```python
from build123d import *

# Parameters (mm, degrees)
SKETCH2_W           = 20
SKETCH2_H           = 10
BOSS_EXTRUDE1_DEPTH = 110
CUT_EXTRUDE1_DEPTH  = 10
SKETCH5_W           = 10
SKETCH5_H           = 60
CUT_EXTRUDE2_DEPTH  = 10
BOSS_EXTRUDE2_DEPTH = 10
FILLET1_R           = 1


with BuildPart() as part:
    # Sketch2 → Boss-Extrude1 (new body)
    with BuildSketch(Plane(origin=(0, 0, 0), x_dir=(1, 0, 0), z_dir=(0, 1, 0))):
        Rectangle(SKETCH2_W, SKETCH2_H)
    extrude(amount=BOSS_EXTRUDE1_DEPTH)

    # Sketch3 → Cut-Extrude1 (cut)
    with BuildSketch(Plane.XY.offset(5)):
        with BuildLine():
            Line((-4.9, 110), (-4.9, 95))
            ThreePointArc((-4.9, 95), (0, 90.1), (4.9, 95))
            Line((4.9, 95), (4.9, 110))
            Line((4.9, 110), (-4.9, 110))
        make_face()
    extrude(amount=-CUT_EXTRUDE1_DEPTH, mode=Mode.SUBTRACT)

    # Sketch5 → Cut-Extrude2 (cut)
    with BuildSketch(Plane.XY.offset(5)):
        with BuildLine():
            Line((-5, 15.05), (5, 15.05))
            ThreePointArc((5, 15.05), (0, 10.05), (-5, 15.05))
        make_face()
        with Locations((0, 45.05)):
            Rectangle(SKETCH5_W, SKETCH5_H)
        with BuildLine():
            ThreePointArc((-5, 75.05), (0, 80.05), (5, 75.05))
            Line((5, 75.05), (-5, 75.05))
        make_face()
    extrude(amount=-CUT_EXTRUDE2_DEPTH, mode=Mode.SUBTRACT)

    # Sketch4 → Boss-Extrude2 (add)
    with BuildSketch(Plane.XY.offset(5)):
        Polygon((-10, 0), (-7.5, 0), (-7.937443318, -5), (-9.33727069, -5), (-10.737534009, -3), (-9.737534009, -3), align=None)
    boss_extrude2 = extrude(amount=-BOSS_EXTRUDE2_DEPTH)

    # Mirror1: Boss-Extrude2 across plane
    add(boss_extrude2.mirror(Plane(origin=(0, 0, 0), x_dir=(0, 0, 1), z_dir=(1, 0, 0))))

    # Fillet1
    fillet1_edges = [part.edges().sort_by_distance(p)[0] for p in [
        (10, 110, 0),
        (-4.9, 110, 0),
        (4.9, 110, 0),
        (-7.5, 0, 0),
        (-10, 110, 0),
        (10, 0, 0),
        (-10, 0, 0),
        (7.5, 0, 0),
    ]]
    fillet(fillet1_edges, radius=FILLET1_R)


solid = part.part
```
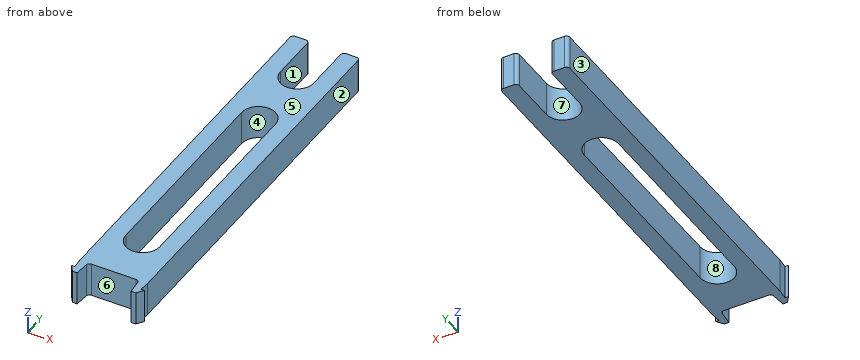
Geometry check sheet. Reference: the model listing, model coordinates, mm. Face numbers are marked on the shaded views. A direction names the side the tool comes from. Give positions to 0.01 mm unless a question says otherwise; leave off trailing zeros. Write each loop counter-clockwise with the first axis right and the second up, starting at its lowest first coordinate (ties: lowest second). Pieces come first, ordered by that corner, then holes.
1) Gauge pin test, flat ends, axial feed: pin 1 (3 mm diameter, centred on y = 56.5, z = -2, fed in from -X); pin 2 (3 mm diameter, centred on y = 58, z = 2, fed in from +X); pin 3 (1.1 mm diameter, centred on x = -10, z = -1.5, fed in from +Y). Record the tip position at first contact, or that the pin passes through.
2) Section check C-C, the plane y = 96. Record the boundary of the cut face in (x, z).
3) Material ranges on L1, parallel to X at y = 19.5, z = -2.25; L2, parallel to X at y = 103, z = -2.5; L3, parallel to X at y = 82, z = -1.5, recorded low to high.
4) Access from +Z, -Z, +X, -X, +Y, -Y to the whole of each face (thin tool, end or side, straight path). Record for the marked faces 1, 2, 3 and 4.
5) Section check B-B, the plane x = 0. Record the boundary of the cut face in (y, z).
6) Release check for a two-part mould opening along Y. For the marked faces 5, 6, 7 and 8 record: pulls with the +Y half, pulls with the -Y half, needs draft (parallel to the pull), parting line crosses it, or undercut.
7) Section check A-A, the plane z = -2.5. Record the boundary of the cut face in (x, y), and give its area (3 significant figures).
Computed:
1. pin 1: stops at x = -10
1. pin 2: stops at x = 10
1. pin 3: stops at y = 109.89
2. outline: (-10, -5) - (-4.9, -5) - (-4.9, 5) - (-10, 5) - close; (4.9, -5) - (10, -5) - (10, 5) - (4.9, 5) - close
3. L1: x = -10 to -5, 5 to 10
3. L2: x = -10 to -4.9, 4.9 to 10
3. L3: x = -10 to 10
4. face 1: +Z, -Z, +Y
4. face 2: +Z, -Z, +X, +Y
4. face 3: +Z, -Z, -X, +Y
4. face 4: +Z, -Z
5. outline: (0, -5) - (10.05, -5) - (10.05, 5) - (0, 5) - close; (80.05, -5) - (90.1, -5) - (90.1, 5) - (80.05, 5) - close
6. face 5: needs draft
6. face 6: pulls with the -Y half
6. face 7: pulls with the +Y half
6. face 8: undercut
7. outline: (-10.74, -3) - (-9.34, -5) - (-7.94, -5) - (-7.58, -0.91) arc R1 cw to (-6.58, 0) - (6.58, 0) arc R1 cw to (7.58, -0.91) - (7.94, -5) - (9.34, -5) - (10.74, -3) - (9.74, -3) - (10, 0) - (10, 109) arc R1 ccw to (9, 110) - (5.9, 110) arc R1 ccw to (4.9, 109) - (4.9, 95) arc R4.9 cw to (-4.9, 95) - (-4.9, 109) arc R1 ccw to (-5.9, 110) - (-9, 110) arc R1 ccw to (-10, 109) - (-10, 0) - (-9.74, -3) - close; hole (-5, 15.05) arc R5 ccw to (5, 15.05) - (5, 75.05) arc R5 ccw to (-5, 75.05) - close
7. area: 1,360 mm2
